The model under review builds one solid part; all positions refer to its coordinate system, in mm. Face numbers are marked on the shaded views. Round coordinates to 2 decimals unless told otherwise and drop trailing zeros. Write each loop counter-clockwise with the first axis right and the second up, starting at its lowest first coordinate (ties: lowest second). Pieces come first, ordered by that corner, then holes. Notation, with made-up numbers: (-4, 1) -> (11, 1) arc R36 cw to (11, 36) -> close; hole circle Ø10 at (54.25, 71). An arc over 180 degrees is marked (long way). Answer as a JSON object with one key per item and string values. Group by question number.
1) We need section C-C, the plane x = 49.5. Write out the cut boundary in (y, z), then the cut area to 3 significant figures.
2) To check wall thickness, follow probe 1 along X at (y, z) = (-3, 1.5); probe 2 along Z at (x, y) = (16, -0.25); probe 3 along Y at (x, z) = (22, 0). State the ranges of each line that lie inside material, in increasing order. Write a range as [from, to].
3) Mouldability with a two-part tool opening along X and no side actions: class the marked faces 1 and 2 as pulls with the +X half, pulls with the -X half, needs draft (parallel to the pull), parting line crosses it, or undercut.
4) Insertion check: pin 1 Ø1.5 at (x, y) = (33, -0.5) entering from -Z; pin 2 Ø4 at (x, y) = (49.5, -3) entering from -Z; pin 3 Ø3 at (x, z) = (22, 1.5) entering from -Y. Each pin has a flat end and moves straight along its axis. Give the tip position at first contact, or say it passes through.
from build123d import *

# Parameters (mm, degrees)
SKETCH1_W     = 18
SKETCH1_H     = 3
SKETCH1_W_2   = 2
SKETCH1_W_3   = 10
SKETCH1_W_4   = 12
FILLET1_R     = 0.2
CHAMFER1_SIZE = 0.3


with BuildPart() as part:
    # Sketch1 → Revolve1 (revolve)
    with BuildSketch(Plane.XY, mode=Mode.PRIVATE) as revolve1_sk:
        Polygon((20, 3), (12, 3), (12, 3.5), (11, 3.5), (11, 3), (0, 3), (0, 0), (20, 0), align=None)
        with Locations((29, 1.5)):
            Rectangle(SKETCH1_W, SKETCH1_H)
        with Locations((39, 1.5)):
            Rectangle(SKETCH1_W_2, SKETCH1_H)
        Polygon((40, 3.5), (40, 3), (40, 0), (48, 0), (48, 3), (41, 3), (41, 3.5), align=None)
        with Locations((53, 1.5)):
            Rectangle(SKETCH1_W_3, SKETCH1_H)
        with Locations((64, 1.5)):
            Rectangle(SKETCH1_W_4, SKETCH1_H)
    revolve(revolve1_sk.sketch.rotate(Axis((0, 0, 0), (1, 0, 0)), 90), axis=Axis((0, 0, 0), (1, 0, 0)))

    # Fillet1
    fillet1_edges = [part.edges().sort_by_distance(p)[0] for p in [
        (11, 0, -3),
        (12, 0, -3),
        (40, 0, -3),
        (41, 0, -3),
    ]]
    fillet(fillet1_edges, radius=FILLET1_R)

    # Chamfer1
    chamfer1_edges = [part.edges().sort_by_distance(p)[0] for p in [
        (0, 0, -3),
        (70, 0, -3),
    ]]
    chamfer(chamfer1_edges, length=CHAMFER1_SIZE)


solid = part.part
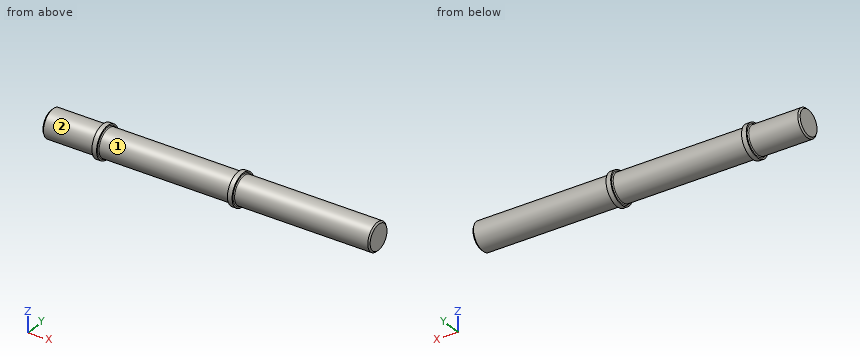
Here are the results:
{
 "1": {"outline": "circle Ø6 at (0, 0)", "area": "28.3 mm^2"},
 "2": {"probe 1": "x = [11, 12], [40, 41]", "probe 2": "z = [-2.99, 2.99]", "probe 3": "y = [-3, 3]"},
 "3": {"face 1": "undercut", "face 2": "needs draft"},
 "4": {"pin 1": "stops at z = -3", "pin 2": "stops at z = -2.83", "pin 3": "stops at y = -3"}
}
